Part model, mm, in its own coordinate system. Face numbers are marked on the shaded views. A direction names the side the tool comes from. Round coordinates to 2 decimals unless told otherwise and drop trailing zeros. Order: outer loops, then holes, each group sorted by start corner. A loop starts at its lowest first (then second) coordinate and runs counter-clockwise, first axis right, second up. Notation, with made-up numbers: M -17,-31.75 L -9,-31.75 A15 cw -9,-22.75 Z; hole C 13,31 d8. An arc over 180 degrees is marked long. One line per question, with ' | ' between items.
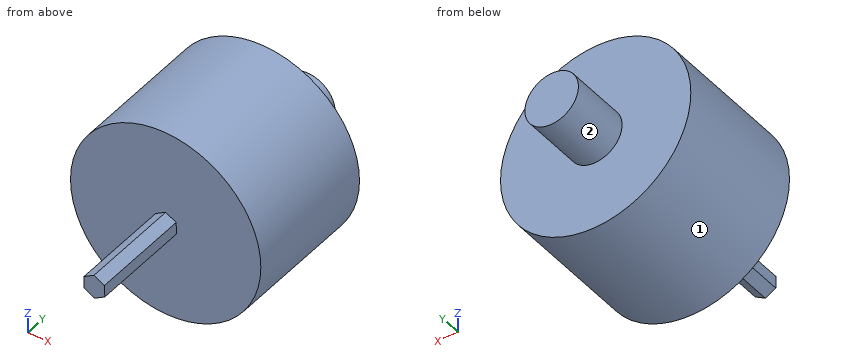
from build123d import *

# Parameters (mm, degrees)
BOSS_EXTRUDE1_DEPTH = 8.305
SKETCH2_R           = 8
BOSS_EXTRUDE2_DEPTH = 11.43
SKETCH3_R           = 2.25
BOSS_EXTRUDE3_DEPTH = 5.06


with BuildPart() as part:
    # Sketch1 → Boss-Extrude1 (new body)
    with BuildSketch(Plane(origin=(0, 0, 0), x_dir=(1, 0, 0), z_dir=(0, 1, 0))):
        Polygon((17.034949463, -13.137071019), (17.914502801, -12.66376429), (17.944383819, -11.665395391), (17.094711499, -11.140333221), (16.215158161, -11.61363995), (16.185277144, -12.612008849), align=None)
    extrude(amount=BOSS_EXTRUDE1_DEPTH)

    # Sketch2 → Boss-Extrude2 (add)
    with BuildSketch(Plane(origin=(0, 8.305, 0), x_dir=(1, 0, 0), z_dir=(0, 1, 0))):
        with Locations((17.034949463, -12.16457984)):
            Circle(SKETCH2_R)
    extrude(amount=BOSS_EXTRUDE2_DEPTH)

    # Sketch3 → Boss-Extrude3 (add)
    with BuildSketch(Plane(origin=(0, 19.735, 0), x_dir=(1, 0, 0), z_dir=(0, 1, 0))):
        with Locations((17.064830481, -12.13870212)):
            Circle(SKETCH3_R)
    extrude(amount=BOSS_EXTRUDE3_DEPTH)


solid = part.part
1) Probe line 1 (Y direction, x = 11.75, z = 14.75) (3 decimals); line 2 (X direction, y = 14.5, z = 12); line 3 (Y direction, x = 15.75, z = 12.5) (3 decimals). List the from-to ranges inside material, lowest first. Write a range as [from, to].
The answers:
line 1: y = [8.305, 19.735] | line 2: x = [9.04, 25.03] | line 3: y = [8.305, 24.795]
2) Which spindle directions (+Z, -Z, +X, -X, +Y, -Y) get a long thin tool onto all of the face, cutting with end or side? Do the marked faces 1 and 2. Say none if no direction does.
The answers:
face 1: +Y, -Y | face 2: +Y
3) Saw through at D-D (y = 21.25). List the corners of the cut face in (x, z), plus the area to 3 significant figures.
The answers:
outline: C 17.06,12.14 d4.5 | area: 15.9 mm²
4) Drop flat-ended pins along their axis: pin 1 (1.5 mm diameter, centred on x = 19.5, z = 16, fed in from +Y) (3 decimals); pin 2 (8 mm diameter, centred on y = 12, z = 17, fed in from -X); pin 3 (1 mm diameter, centred on x = 13.5, y = 13, fed in from -Z); pin 4 (2 mm diameter, centred on x = 23, y = 5.5, fed in from +Z). Give the stop position or say it passes through.
The answers:
pin 1: stops at y = 19.735 | pin 2: stops at x = 9.08 | pin 3: stops at z = 4.76 | pin 4: passes through
5) Saw through at B-B (y = 4.5). List the corners of the cut face in (x, z).
The answers:
outline: M 16.19,12.61 L 16.22,11.61 L 17.09,11.14 L 17.94,11.67 L 17.91,12.66 L 17.03,13.14 Z
6) Saw through at C-C (x = 19). List the corners of the cut face in (y, z) (3 decimals).
The answers:
outline: M 8.305,4.41 L 19.735,4.41 L 19.735,10.991 L 24.795,10.991 L 24.795,13.287 L 19.735,13.287 L 19.735,19.919 L 8.305,19.919 Z
7) Saw through at A-A (z = 14). List the corners of the cut face in (x, y) (3 decimals), plus the area to 3 significant figures.
The answers:
outline: M 9.248,8.305 L 24.822,8.305 L 24.822,19.735 L 18.329,19.735 L 18.329,24.795 L 15.801,24.795 L 15.801,19.735 L 9.248,19.735 Z | area: 191 mm²
